Geometry check sheet. Reference: drawing and pictorial views, mm from the part's lowest x, y, z. Give positions to 0.01 mm unless a question says otherwise; leave off trailing zeros. Write each loop counter-clockwise with the first axis right and the second up, starting at its lowest first coordinate (ties: lowest second). Pieces come first, ordered by that corner, then holes. Notation, with made-up numbers: (36, 26.25) -> (46, 26.25) arc R28 cw to (46, 62.25) -> close; hole circle Ø7 at (76, 19). An arc over 180 degrees is marked (long way). Use a Markdown table: item, result. Add a question column.
1. Cross-section at C-C (x = 657.5). Enter the section's corners in (y, z), then the cut area to 3 significant figures.
2. Scan lines: probe 1 along X at (y, z) = (641, 25.75); probe 2 along Y at (x, z) = (510, 20); probe 3 along X at (y, z) = (1078, 4.25). Record each from-to range of solid material in increasing order. Write a range as [from, to].
3. Cross-section at A-A (y = 904.5). Enter the section's corners in (x, z).
4. Gauge pin test, flat ends, axial feed: P1, Ø1, axis at y = 335, z = 10.5, coming from the +X side; P2, Ø4.5, axis at y = 783, z = 24, coming from the +X side; P3, Ø16.5, axis at x = 864.5, y = 411, coming from the -Z side. Record the tip position at first contact, or that the pin passes through.
5. Cross-section at B-B (z = 22). Enter the section's corners in (x, y).
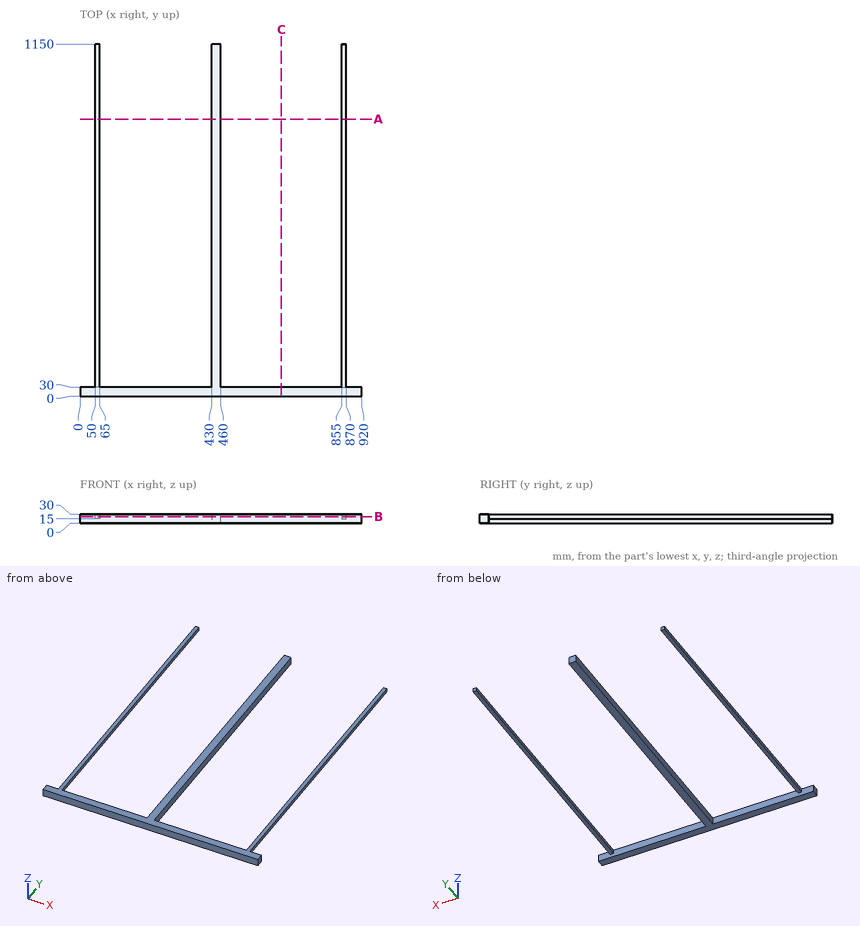
Worked answers:
| question | item | result |
|---|---|---|
| 1 | outline | (0, 0) -> (30, 0) -> (30, 30) -> (0, 30) -> close |
| 1 | area | 900 mm² |
| 2 | probe 1 | x = [50, 65], [430, 460], [855, 870] |
| 2 | probe 2 | y = [0, 30] |
| 2 | probe 3 | x = [430, 460] |
| 3 | outline | (50, 15) -> (65, 15) -> (65, 30) -> (50, 30) -> close; (430, 0) -> (460, 0) -> (460, 30) -> (430, 30) -> close; (855, 15) -> (870, 15) -> (870, 30) -> (855, 30) -> close |
| 4 | P1 | stops at x = 460 |
| 4 | P2 | stops at x = 870 |
| 4 | P3 | stops at z = 15 |
| 5 | outline | (0, 0) -> (920, 0) -> (920, 30) -> (870, 30) -> (870, 1150) -> (855, 1150) -> (855, 30) -> (460, 30) -> (460, 1150) -> (430, 1150) -> (430, 30) -> (65, 30) -> (65, 1150) -> (50, 1150) -> (50, 30) -> (0, 30) -> close |
